Part model, mm, in its own coordinate system. Round coordinates to 2 decimals unless told otherwise and drop trailing zeros. Loops run counter-clockwise (first coordinate to the right, second up) from the corner with the lowest first, then second, coordinate; pieces in that order, holes last. Notation, with made-up numbers: (80, 82.5) -> (107, 82.5) arc R20 cw to (107, 118.5) -> close; hole circle Ø11 at (63.25, 44.5). An arc over 180 degrees is marked (long way). Use a Markdown table: item, result. Add a question column.
Item 1: Flat gauge pins, fed straight in: pin 1 (5 mm diameter, centred on y = 61.5, z = 10.5, fed in from -X); pin 2 (2 mm diameter, centred on x = -117, z = 8, fed in from +Y); pin 3 (6.5 mm diameter, centred on x = -180.01, y = 0, fed in from -Z). Where does each tip first touch, or does it go through?
Item 2: Cut at A-A, the plane y = 0. List the corners of the cut face in (x, z).
Item 3: Probe line 1 (Y direction, x = -115, z = 1); line 2 (Y direction, x = -178.5, z = 6.5); line 3 (X direction, y = 69.5, z = 6.75). List the from-to ranges inside material, lowest first. Write a range as [from, to].
Item 4: Cut at D-D, the plane x = -69.5. List the corners of the cut face in (y, z).
Item 5: Cut at B-B, the plane z = 7. List the corners of the cut face in (x, y).
Item 6: Cut at C-C, the plane y = 23.5. List the corners of the cut face in (x, z), plus the area to 3 significant figures.
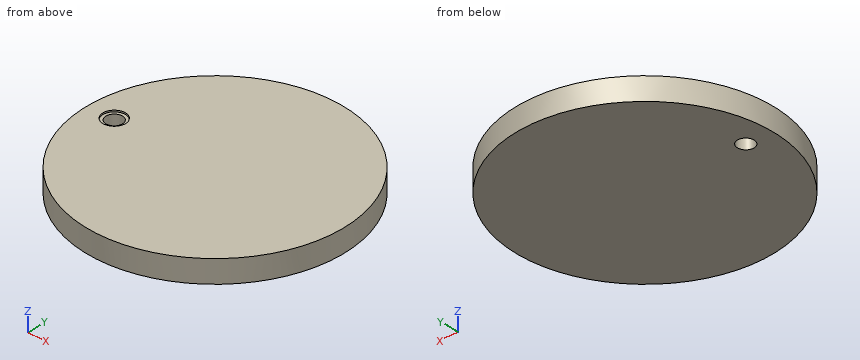
```python
from build123d import *

# Parameters (mm, degrees)
ESQUISSE1_R             = 85
BOSS_EXTRU_1_DEPTH      = 15
ESQUISSE2_R             = 7.5
ENL_V_MAT_EXTRU_1_DEPTH = 1
ESQUISSE4_R             = 5.5
ENL_V_MAT_EXTRU_2_DEPTH = 15


with BuildPart() as part:
    # Esquisse1 → Boss.-Extru.1 (new body)
    with BuildSketch(Plane.XY):
        with Locations((-112.573673301, 0)):
            Circle(ESQUISSE1_R)
    extrude(amount=BOSS_EXTRU_1_DEPTH)

    # Esquisse2 → Enlèv. mat.-Extru.1 (cut)
    with BuildSketch(Plane.XY.offset(15)):
        with Locations((-180.019561977, 0)):
            Circle(ESQUISSE2_R)
    extrude(amount=-ENL_V_MAT_EXTRU_1_DEPTH, mode=Mode.SUBTRACT)

    # Esquisse4 → Enlèv. mat.-Extru.2 (cut)
    with BuildSketch(Plane.XY.offset(14)):
        with Locations((-180.010590856, 0)):
            Circle(ESQUISSE4_R)
    extrude(amount=-ENL_V_MAT_EXTRU_2_DEPTH, mode=Mode.SUBTRACT)


solid = part.part
```
A:
| question | item | result |
|---|---|---|
| 1 | pin 1 | stops at x = -173.76 |
| 1 | pin 2 | stops at y = 84.93 |
| 1 | pin 3 | passes through |
| 2 | outline | (-197.57, 0) -> (-185.51, 0) -> (-185.51, 14) -> (-187.52, 14) -> (-187.52, 15) -> (-197.57, 15) -> close; (-174.51, 0) -> (-27.57, 0) -> (-27.57, 15) -> (-172.52, 15) -> (-172.52, 14) -> (-174.51, 14) -> close |
| 3 | line 1 | y = [-84.97, 84.97] |
| 3 | line 2 | y = [-53.65, -5.29], [5.29, 53.65] |
| 3 | line 3 | x = [-161.51, -63.64] |
| 4 | outline | (-73.28, 0) -> (73.28, 0) -> (73.28, 15) -> (-73.28, 15) -> close |
| 5 | outline | circle Ø170 at (-112.57, 0); hole circle Ø11 at (-180.01, 0) |
| 6 | outline | (-194.26, 0) -> (-30.89, 0) -> (-30.89, 15) -> (-194.26, 15) -> close |
| 6 | area | 2,450 mm^2 |
